```python
from build123d import *

# Parameters (mm, degrees)
F1_DEPTH     = 19
F2_R         = 5
F3_T1_DEPTH  = 104.8421979693
F3_T3_DEPTH  = 119.7500710634
F3_T5_DEPTH  = 119.7500710634
F3_T7_DEPTH  = 119.7500710634
F3_T9_DEPTH  = 104.8421979693
F3_T11_DEPTH = 20.0196827351
F3_T16_DEPTH = 5
F3_T22_DEPTH = 5


# Not quite as in the source:
# - a fillet or chamfer that OpenCascade refuses, or shapes differently, is made with other operations: its cross-section is extruded or revolved along the edge and cut away or added


with BuildPart() as f1:
    # F0 (on Top) → F1 (new body)
    with BuildSketch(Plane.XY):
        Polygon((41.3957443257, 101.0370281819), (-53.1841051002, 95.3600528356), (-107.7152386276, 17.8750127135), (-81.134600478, -73.0702765657), (6.5420466758, -108.9921572289), (89.2923992493, -62.8407204639), (104.8037539551, 30.6310605275), align=None)
    extrude(amount=F1_DEPTH)

    # F2
    f2_edges = [f1.edges().sort_by_distance(p)[0] for p in [
        (-94.42492, -27.597632, 19),
        (-37.296277, -91.031217, 19),
    ]]
    fillet(f2_edges, radius=F2_R)

    # F3: fillet of radius 5 on 7 edges, made by hand

    # F3_s2 → F3_t1 (cut)
    with BuildSketch(Plane(origin=(-39.2722507137, -21.9028770158, 0), x_dir=(0, 0, 1), z_dir=(0.8733539896, 0.4870860385, 0))):
        with BuildLine():
            ThreePointArc((19, 93.3752749449), (17.5355339059, 96.9108088508), (14, 98.3752749449))
            Line((14, 98.3752749449), (19, 98.3752749449))
            Line((19, 98.3752749449), (19, 93.3752749449))
        make_face()
    extrude(amount=F3_T1_DEPTH, mode=Mode.SUBTRACT)

    # F3_s4 → F3_t3 (cut)
    with BuildSketch(Plane(origin=(-9.8020286817, -59.067250771, 0), x_dir=(0, 0, 1), z_dir=(0.1637081063, 0.986508822, 0))):
        with BuildLine():
            ThreePointArc((19, 93.3752749449), (17.5355339059, 96.9108088508), (14, 98.3752749449))
            Line((14, 98.3752749449), (19, 98.3752749449))
            Line((19, 98.3752749449), (19, 93.3752749449))
        make_face()
    extrude(amount=F3_T3_DEPTH, mode=Mode.SUBTRACT)

    # F3_s6 → F3_t5 (cut)
    with BuildSketch(Plane(origin=(40.0691713151, -44.4913630949, 0), x_dir=(0, 0, 1), z_dir=(-0.66921332, 0.7430703414, 0))):
        with BuildLine():
            ThreePointArc((19, 93.3752749449), (17.5355339059, 96.9108088508), (14, 98.3752749449))
            Line((14, 98.3752749449), (19, 98.3752749449))
            Line((19, 98.3752749449), (19, 93.3752749449))
        make_face()
    extrude(amount=F3_T5_DEPTH, mode=Mode.SUBTRACT)

    # F3_s8 → F3_t7 (cut)
    with BuildSketch(Plane(origin=(59.7674680494, 3.58742845, 0), x_dir=(0, 0, 1), z_dir=(-0.9982034669, -0.0599152621, 0))):
        with BuildLine():
            ThreePointArc((19, 93.3752749449), (17.5355339059, 96.9108088508), (14, 98.3752749449))
            Line((14, 98.3752749449), (19, 98.3752749449))
            Line((19, 98.3752749449), (19, 93.3752749449))
        make_face()
    extrude(amount=F3_T7_DEPTH, mode=Mode.SUBTRACT)

    # F3_s10 → F3_t9 (cut)
    with BuildSketch(Plane(origin=(34.4596423084, 48.9648132019, 0), x_dir=(0, 0, 1), z_dir=(-0.5755260436, -0.8177834513, 0))):
        with BuildLine():
            ThreePointArc((14, 98.3752749449), (17.5355339059, 96.9108088508), (19, 93.3752749449))
            Line((19, 93.3752749449), (19, 98.3752749449))
            Line((19, 98.3752749449), (14, 98.3752749449))
        make_face()
    extrude(amount=F3_T9_DEPTH, mode=Mode.SUBTRACT)

    # F3_s12 → F3_t11 (cut)
    with BuildSketch(Plane.XY.offset(-6.0196827351)):
        with BuildLine():
            ThreePointArc((-106.3294449524, 19.8441314825), (-107.1730718062, 17.7850417962), (-107.0397478053, 15.5638301188))
            Line((-107.0397478053, 15.5638301188), (-107.7152386276, 17.8750127135))
            Line((-107.7152386276, 17.8750127135), (-106.3294449524, 19.8441314825))
        make_face()
        with BuildLine():
            ThreePointArc((4.3139297226, -108.0792784419), (6.5091183669, -108.443563249), (8.6449722488, -107.8193158622))
            Line((8.6449722488, -107.8193158622), (6.5420466758, -108.9921572289))
            Line((6.5420466758, -108.9921572289), (4.3139297226, -108.0792784419))
        make_face()
    extrude(amount=F3_T11_DEPTH, mode=Mode.SUBTRACT)


with BuildPart() as f3_tool14:
    # F3_s15 → F3_t16 (new body)
    with BuildSketch(Plane.XY.offset(14)):
        Polygon((6.2095420561, -103.4525459145), (4.3139297226, -108.0792784419), (6.5420466758, -108.9921572289), (8.6449722488, -107.8193158622), align=None)
    extrude(amount=F3_T16_DEPTH)

    # F3_s17 → F3_t18 (revolve, cut)
    with BuildSketch(Plane(origin=(6.2095420561, -103.4525459145, 14), x_dir=(-0.0599152621, 0.9982034669, 0), z_dir=(0.9982034669, 0.0599152621, 0))):
        with BuildLine():
            ThreePointArc((0, -5), (5, 0), (0, 5))
            Line((0, 5), (0, -5))
        make_face()
    revolve(axis=Axis((6.2095420561, -103.4525459145, 14), (0, 0, 1)), mode=Mode.SUBTRACT)


with BuildPart() as f1_1:
    add(f1.part)

    # F3_t13: cut F3_tool14
    add(f3_tool14.part, mode=Mode.SUBTRACT)


with BuildPart() as f3_tool20:
    # F3_s21 → F3_t22 (new body)
    with BuildSketch(Plane.XY.offset(14)):
        Polygon((-102.240527696, 16.9665012646), (-106.3294449524, 19.8441314825), (-107.7152386276, 17.8750127135), (-107.0397478053, 15.5638301188), align=None)
    extrude(amount=F3_T22_DEPTH)

    # F3_s23 → F3_t24 (revolve, cut)
    with BuildSketch(Plane(origin=(-102.240527696, 16.9665012646, 14), x_dir=(0.986508822, -0.1637081063, 0), z_dir=(-0.1637081063, -0.986508822, 0))):
        with BuildLine():
            ThreePointArc((0, -5), (5, 0), (0, 5))
            Line((0, 5), (0, -5))
        make_face()
    revolve(axis=Axis((-102.240527696, 16.9665012646, 14), (0, 0, 1)), mode=Mode.SUBTRACT)


with BuildPart() as f1_2:
    add(f1_1.part)

    # F3_t19: cut F3_tool20
    add(f3_tool20.part, mode=Mode.SUBTRACT)


solid = f1_2.part
```
Geometry check sheet. Reference: the model listing, model coordinates, mm. Coordinates: 2 decimals unless noted, no trailing zeros. Order: outer loops, then holes, each group sorted by start corner. A loop starts at its lowest first (then second) coordinate and runs counter-clockwise, first axis right, second up. Notation, with made-up numbers: (47, 37.25) - (83, 37.25) arc R10 cw to (83, 56.25) - close; hole circle Ø1 at (-24.75, 63.25). An arc over 180 degrees is marked (long way). Answer as a JSON object with one key per item and string values. Group by question number.
Item 1: Scan lines: probe 1 along Y at (x, z) = (27.5, 10); probe 2 along X at (y, z) = (-90, 13); probe 3 along X at (y, z) = (68.5, 13.25). Record each from-to range of solid material in increasing order.
Item 2: Depth check by flat-ended pin: pin 1 Ø3 at (y, z) = (9, 8) entering from -X; pin 2 Ø1.5 at (x, z) = (68, 6) entering from +Y; pin 3 Ø8 at (y, z) = (71.5, 14) entering from +X. Enter the tip coordinate at first touch or a pass-through.
Item 3: Sectioned sample at A-A, the plane z = 5.25. Record the cut outline in (x, y).
Resolved:
{
 "1": {"probe 1": "-97.3 to 100.2", "probe 2": "-39.81 to 40.6", "probe 3": "-72.09 to 70.7"},
 "2": {"pin 1": "x = -105.56", "pin 2": "y = 72.33", "pin 3": "x = 71.6"},
 "3": {"outline": "(-107.04, 15.56) - (-81.13, -73.07) - (4.31, -108.08) arc R5 ccw to (8.64, -107.82) - (89.29, -62.84) - (104.8, 30.63) - (41.4, 101.04) - (-53.18, 95.36) - (-106.33, 19.84) arc R5 ccw to start"}
}
